The listing builds one solid part. Answer for the finished solid, in the listing's coordinates (mm). A direction names the side the tool comes from. Round coordinates to 2 decimals unless told otherwise and drop trailing zeros. Write each loop counter-clockwise with the first axis right and the second up, starting at its lowest first coordinate (ties: lowest second). Pieces come first, ordered by that corner, then holes. Notation, with made-up numbers: (23.5, 56) - (66.5, 56) arc R11 cw to (66.5, 63) - close; hole circle Ø4 at (-8.75, 43.25). An arc over 180 degrees is marked (long way). Use a Markdown table: item, result. Add a question column.
1) Determine the mould class of faces 4 (the cylindrical face through (14.85, -4.06, 7.89)), 5 (the flat face through (13, -8, 10)), 6 (the cylindrical face through (0.3, -4.1, 2.8)) for opening direction Z: +Z half, -Z half, draft (parallel to the pull), parting line (faces both ways), or undercut.
2) Each of these flat-tipped pins is pushed along its axis until it touches: P1, Ø1.8, axis at x = 13.5, y = -3.5, coming from the +Z side; P2, Ø1.5, axis at y = -3, z = 16, coming from the +X side; P3, Ø5, axis at y = -3, z = 9, coming from the +X side. Where does it stop, or does it pass through?
3) A cutting plane is placed at B-B (y = 0.75). Give the vertices of the cut face in (x, z) (3 decimals), then the cut area to 3 significant figures.
4) A tool of negligible diameter and unlimited length cuts with its end or side. For faces 1 (the flat face through (0, 1.5, 0)), 2 (the flat face through (0.267, -3.32, 6.88)), 3 (the cylindrical face through (-16.24, -3.55, -9.52)), from which of +Z, -Z, +X, -X, +Y, -Y can it reach the whole face along a straight path? Write none if from no direction.
5) Find the intervals of material crossed by probe 1 along Y at (x, z) = (-11.5, -7); probe 2 along X at (y, z) = (-1.75, 2.5); probe 3 along Z at (x, y) = (8, -0.5), in increasing order. Write a range as from..to.
6) A cutting plane is placed at D-D (z = 15.5). Give the vertices of the cut face in (x, y), then the cut area to 3 significant figures.
7) A cutting plane is placed at A-A (y = -2.25). Give the vertices of the cut face in (x, z) (3 decimals), then the cut area to 3 significant figures.
8) A cutting plane is placed at C-C (x = 11). Give the vertices of the cut face in (y, z), then the cut area to 3 significant figures.
```python
from build123d import *

# Parameters (mm, degrees)
SKETCH1_R           = 22.5
SKETCH1_R_2         = 4.75
SKETCH1_R_3         = 10
SKETCH1_R_4         = 2.55
SKETCH1_R_5         = 9.761790251
SKETCH1_R_6         = 9
BOSS_EXTRUDE1_DEPTH = 1.5
BOSS_EXTRUDE2_START = -8
SKETCH1_3_R         = 9.761790251
SKETCH1_3_R_2       = 9
SKETCH1_3_R_3       = 2.55
BOSS_EXTRUDE2_DEPTH = 8
FILLET1_R           = 1


with BuildPart() as part:
    # Sketch1 → Boss-Extrude1 (new body)
    # profile 1 of 11: a face of its own
    with BuildSketch(Plane(origin=(0, 0, 0), x_dir=(1, 0, 0), z_dir=(0, 1, 0))):
        with Locations(Location((0, 0, 0), (0, 0, 270))):
            Circle(SKETCH1_R)
        with Locations((-13.75, 8.96333732)):
            Circle(SKETCH1_R_2, mode=Mode.SUBTRACT)
        with Locations((6.25, -10.53666268)):
            Circle(SKETCH1_R_3, mode=Mode.SUBTRACT)
    # profile 2 of 11: a face of its own
    with BuildSketch(Plane(origin=(0, 0, 0), x_dir=(1, 0, 0), z_dir=(0, 1, 0))):
        with Locations((-13.75, 8.96333732)):
            Circle(SKETCH1_R_2)
        with Locations((-13.75, 8.96333732)):
            Circle(SKETCH1_R_4, mode=Mode.SUBTRACT)
    # profile 3 of 11: a face of its own
    with BuildSketch(Plane(origin=(0, 0, 0), x_dir=(1, 0, 0), z_dir=(0, 1, 0))):
        with Locations((-13.75, 8.96333732)):
            Circle(SKETCH1_R_4)
    # profile 4 of 11: a face of its own
    with BuildSketch(Plane(origin=(0, 0, 0), x_dir=(1, 0, 0), z_dir=(0, 1, 0))):
        with Locations((6.25, -10.53666268)):
            Circle(SKETCH1_R_3)
        with Locations((6.25, -10.53666268)):
            Circle(SKETCH1_R_5, mode=Mode.SUBTRACT)
    # profile 5 of 11: a face of its own
    with BuildSketch(Plane(origin=(0, 0, 0), x_dir=(1, 0, 0), z_dir=(0, 1, 0))):
        with Locations((6.25, -10.53666268)):
            Circle(SKETCH1_R_5)
        with Locations((6.25, -10.53666268)):
            Circle(SKETCH1_R_6, mode=Mode.SUBTRACT)
    # profile 6 of 11: a face of its own
    with BuildSketch(Plane(origin=(0, 0, 0), x_dir=(1, 0, 0), z_dir=(0, 1, 0))):
        with BuildLine():
            ThreePointArc((-1.233314774, -5.53666268), (-1.6730161, -6.267492282), (-2.041561976, -7.03666268))
            Line((-2.041561976, -7.03666268), (0.266685226, -7.03666268))
            Line((0.266685226, -7.03666268), (0.266685226, -5.53666268))
            Line((0.266685226, -5.53666268), (-1.233314774, -5.53666268))
        make_face()
    # profile 7 of 11: a face of its own
    with BuildSketch(Plane(origin=(0, 0, 0), x_dir=(1, 0, 0), z_dir=(0, 1, 0))):
        with BuildLine():
            ThreePointArc((-2.041561976, -7.03666268), (-2.346986264, -7.873614205), (-2.568163074, -8.73666268))
            Line((-2.568163074, -8.73666268), (0.266685226, -8.73666268))
            Line((0.266685226, -8.73666268), (0.266685226, -7.03666268))
            Line((0.266685226, -7.03666268), (-2.041561976, -7.03666268))
        make_face()
    # profile 8 of 11: a face of its own
    with BuildSketch(Plane(origin=(0, 0, 0), x_dir=(1, 0, 0), z_dir=(0, 1, 0))):
        with BuildLine():
            Line((0.266685226, -8.73666268), (-2.568163074, -8.73666268))
            ThreePointArc((-2.568163074, -8.73666268), (-2.688102836, -9.482946541), (-2.74499861, -10.23666268))
            Line((-2.74499861, -10.23666268), (0.266685226, -10.23666268))
            Line((0.266685226, -10.23666268), (0.266685226, -8.73666268))
        make_face()
    # profile 9 of 11: a face of its own
    with BuildSketch(Plane(origin=(0, 0, 0), x_dir=(1, 0, 0), z_dir=(0, 1, 0))):
        with BuildLine():
            ThreePointArc((14.541561976, -7.03666268), (14.1730161, -6.267492282), (13.733314774, -5.53666268))
            Line((13.733314774, -5.53666268), (12.233314774, -5.53666268))
            Line((12.233314774, -5.53666268), (12.233314774, -7.03666268))
            Line((12.233314774, -7.03666268), (14.541561976, -7.03666268))
        make_face()
    # profile 10 of 11: a face of its own
    with BuildSketch(Plane(origin=(0, 0, 0), x_dir=(1, 0, 0), z_dir=(0, 1, 0))):
        with BuildLine():
            ThreePointArc((15.068163074, -8.73666268), (14.846986264, -7.873614205), (14.541561976, -7.03666268))
            Line((14.541561976, -7.03666268), (12.233314774, -7.03666268))
            Line((12.233314774, -7.03666268), (12.233314774, -8.73666268))
            Line((12.233314774, -8.73666268), (15.068163074, -8.73666268))
        make_face()
    # profile 11 of 11: a face of its own
    with BuildSketch(Plane(origin=(0, 0, 0), x_dir=(1, 0, 0), z_dir=(0, 1, 0))):
        with BuildLine():
            Line((12.233314774, -10.23666268), (15.24499861, -10.23666268))
            ThreePointArc((15.24499861, -10.23666268), (15.188102836, -9.482946541), (15.068163074, -8.73666268))
            Line((15.068163074, -8.73666268), (12.233314774, -8.73666268))
            Line((12.233314774, -8.73666268), (12.233314774, -10.23666268))
        make_face()
    extrude(amount=BOSS_EXTRUDE1_DEPTH)

    # Sketch1_3 → Boss-Extrude2 (add)
    # profile 1 of 6: a face of its own
    with BuildSketch(Plane(origin=(0, 0, 0), x_dir=(1, 0, 0), z_dir=(0, 1, 0)).offset(BOSS_EXTRUDE2_START)):
        with Locations(Location((6.25, -10.53666268, 0), (0, 0, 270))):
            Circle(SKETCH1_3_R)
        with Locations((6.25, -10.53666268)):
            Circle(SKETCH1_3_R_2, mode=Mode.SUBTRACT)
    # profile 2 of 6: a face of its own
    with BuildSketch(Plane(origin=(0, 0, 0), x_dir=(1, 0, 0), z_dir=(0, 1, 0)).offset(BOSS_EXTRUDE2_START)):
        with Locations(Location((-13.75, 8.96333732, 0), (0, 0, 270))):
            Circle(SKETCH1_3_R_3)
    # profile 3 of 6: a face of its own
    with BuildSketch(Plane(origin=(0, 0, 0), x_dir=(1, 0, 0), z_dir=(0, 1, 0)).offset(BOSS_EXTRUDE2_START)):
        with BuildLine():
            ThreePointArc((14.541561976, -7.03666268), (14.1730161, -6.267492282), (13.733314774, -5.53666268))
            Line((13.733314774, -5.53666268), (12.233314774, -5.53666268))
            Line((12.233314774, -5.53666268), (12.233314774, -7.03666268))
            Line((12.233314774, -7.03666268), (14.541561976, -7.03666268))
        make_face()
    # profile 4 of 6: a face of its own
    with BuildSketch(Plane(origin=(0, 0, 0), x_dir=(1, 0, 0), z_dir=(0, 1, 0)).offset(BOSS_EXTRUDE2_START)):
        with BuildLine():
            Line((12.233314774, -10.23666268), (15.24499861, -10.23666268))
            ThreePointArc((15.24499861, -10.23666268), (15.188102836, -9.482946541), (15.068163074, -8.73666268))
            Line((15.068163074, -8.73666268), (12.233314774, -8.73666268))
            Line((12.233314774, -8.73666268), (12.233314774, -10.23666268))
        make_face()
    # profile 5 of 6: a face of its own
    with BuildSketch(Plane(origin=(0, 0, 0), x_dir=(1, 0, 0), z_dir=(0, 1, 0)).offset(BOSS_EXTRUDE2_START)):
        with BuildLine():
            Line((0.266685226, -8.73666268), (-2.568163074, -8.73666268))
            ThreePointArc((-2.568163074, -8.73666268), (-2.688102836, -9.482946541), (-2.74499861, -10.23666268))
            Line((-2.74499861, -10.23666268), (0.266685226, -10.23666268))
            Line((0.266685226, -10.23666268), (0.266685226, -8.73666268))
        make_face()
    # profile 6 of 6: a face of its own
    with BuildSketch(Plane(origin=(0, 0, 0), x_dir=(1, 0, 0), z_dir=(0, 1, 0)).offset(BOSS_EXTRUDE2_START)):
        with BuildLine():
            ThreePointArc((-1.233314774, -5.53666268), (-1.6730161, -6.267492282), (-2.041561976, -7.03666268))
            Line((-2.041561976, -7.03666268), (0.266685226, -7.03666268))
            Line((0.266685226, -7.03666268), (0.266685226, -5.53666268))
            Line((0.266685226, -5.53666268), (-1.233314774, -5.53666268))
        make_face()
    extrude(amount=BOSS_EXTRUDE2_DEPTH)

    # Fillet1
    fillet1_edges = [part.edges().sort_by_distance(p)[0] for p in [
        (-13.75, -8, -11.51333732),
    ]]
    fillet(fillet1_edges, radius=FILLET1_R)


solid = part.part
```
Entries:
| question | item | result |
|---|---|---|
| 1 | face 4 | undercut |
| 1 | face 5 | draft |
| 1 | face 6 | parting line |
| 2 | P1 | stops at z = 17.95 |
| 2 | P2 | stops at x = 14.8 |
| 2 | P3 | stops at x = 16.01 |
| 3 | outline | circle Ø45 at (0, 0); hole (-2.745, 10.237) - (0.267, 10.237) - (0.267, 5.537) - (-1.233, 5.537) arc R9 ccw to (13.733, 5.537) - (12.233, 5.537) - (12.233, 10.237) - (15.245, 10.237) arc R9 ccw (long way) to start |
| 3 | area | 1,360 mm² |
| 4 | face 1 | +Z, -Z, +X, -X, +Y |
| 4 | face 2 | +Y, -Y |
| 4 | face 3 | -Y |
| 5 | probe 1 | y = 0..1.5 |
| 5 | probe 2 | x = 0.71..2.2, 10.3..11.79 |
| 5 | probe 3 | z = 0.93..1.71, 19.36..20.14 |
| 6 | outline | (-16.31, 0) - (-2.16, 0) - (-2.16, -8) - (-1.26, -8) - (-1.26, 1.5) - (-16.31, 1.5) - close; (13.76, -8) - (14.66, -8) - (14.66, 0) - (16.31, 0) - (16.31, 1.5) - (13.76, 1.5) - close |
| 6 | area | 40.8 mm² |
| 7 | outline | circle Ø5.1 at (-13.75, -8.963); circle Ø19.524 at (6.25, 10.537); hole (-2.745, 10.237) - (0.267, 10.237) - (0.267, 8.737) - (-2.568, 8.737) arc R9 ccw to (-2.042, 7.037) - (0.267, 7.037) - (0.267, 5.537) - (-1.233, 5.537) arc R9 ccw to (13.733, 5.537) - (12.233, 5.537) - (12.233, 7.037) - (14.542, 7.037) arc R9 ccw to (15.068, 8.737) - (12.233, 8.737) - (12.233, 10.237) - (15.245, 10.237) arc R9 ccw (long way) to start |
| 7 | area | 80.0 mm² |
| 8 | outline | (-8, 2.01) - (0, 2.01) - (0, -19.63) - (1.5, -19.63) - (1.5, 2.89) - (-8, 2.89) - close; (-8, 18.18) - (1.5, 18.18) - (1.5, 19.63) - (0, 19.63) - (0, 19.06) - (-8, 19.06) - close |
| 8 | area | 50.1 mm² |
